Part print with two shaded views. Sizes in mm from the minimum x, y, z corner. A direction names the side the tool comes from. Coordinates: 2 decimals unless noted, no trailing zeros. Loops run counter-clockwise (first coordinate to the right, second up) from the corner with the lowest first, then second, coordinate; pieces in that order, holes last. Notation, with made-up numbers: (13.5, 43) -> (67.5, 43) arc R14 cw to (67.5, 48) -> close; hole circle Ø6 at (-3.5, 82.25). An arc over 180 degrees is marked (long way). Return JSON: item names as keys, results as strings. Group by question number.
(1) Saw through at B-B on z = 162. Write the cut outline in (x, y).
(2) Flat gauge pins, fed straight in: pin 1 Ø4 at (x, y) = (208, 21.5) entering from +Z; pin 2 Ø0.7 at (y, z) = (1, 60) entering from -X; pin 3 Ø6 at (y, z) = (151.5, 230.5) entering from -X. Where does each tip first touch, or does it go through?
(3) Saw through at A-A on y = 153. Write the cut outline in (x, z), then the cut area to 3 significant figures.
(4) Probe L1, parallel to Z at x = 310, y = 148.5; L2, parallel to Z at x = 160.5, y = 121; L3, parallel to X at y = 87, z = 85. List the from-to ranges inside material, lowest first.
(5) Saw through at D-D on z = 83. Write the cut outline in (x, y).
(6) Saw through at C-C on x = 152.5. Write the cut outline in (y, z).
(7) Mould opens along Y. For the marked faces 3, 4, 5 and 6 say: pulls with the +Y half, pulls with the -Y half, needs draft (parallel to the pull), parting line crosses it, or undercut.
(8) Tool access for the marked faces 1 and 2: list every direction of +Z, -Z, +X, -X, +Y, -Y with a clear straight run to the whole face (end or side of a thin tool).
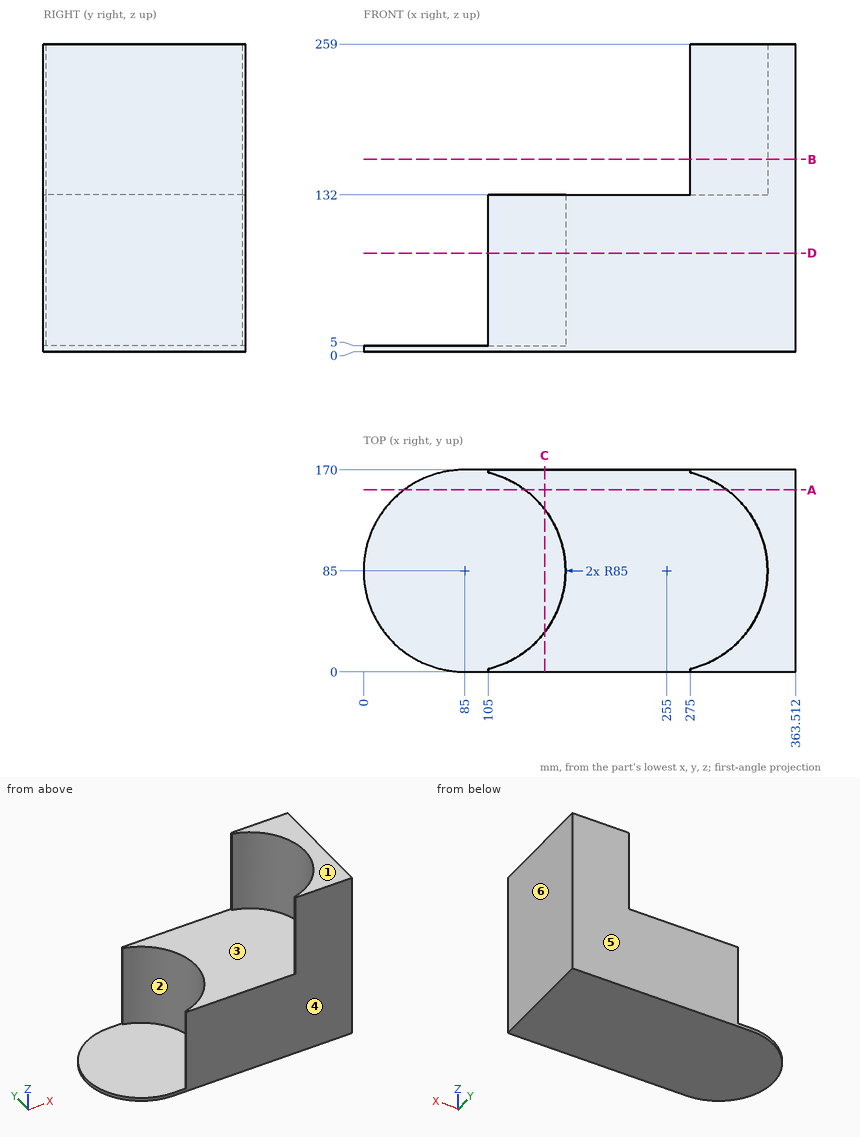
Geometry results:
{
 "1": {"outline": "(275, 0) -> (363.51, 0) -> (363.51, 170) -> (275, 170) -> (275, 167.61) arc R85 cw to (275, 2.39) -> close"},
 "2": {"pin 1": "z = 132", "pin 2": "x = 105", "pin 3": "x = 303.94"},
 "3": {"outline": "(34, 0) -> (363.51, 0) -> (363.51, 259) -> (306, 259) -> (306, 132) -> (136, 132) -> (136, 5) -> (34, 5) -> close", "area": "37,800 mm²"},
 "4": {"L1": "0 to 132", "L2": "0 to 5", "L3": "169.98 to 363.51"},
 "5": {"outline": "(105, 0) -> (363.51, 0) -> (363.51, 170) -> (105, 170) -> (105, 167.61) arc R85 cw to (105, 2.39) -> close"},
 "6": {"outline": "(0, 0) -> (170, 0) -> (170, 132) -> (136.66, 132) -> (136.66, 5) -> (33.34, 5) -> (33.34, 132) -> (0, 132) -> close"},
 "7": {"face 3": "undercut", "face 4": "pulls with the -Y half", "face 5": "pulls with the +Y half", "face 6": "needs draft"},
 "8": {"face 1": "+Z, +X, -X, +Y, -Y", "face 2": "+Z, -X"}
}
